Verification items for the finished model (mm, model axes). Face numbers are marked on the shaded views. A direction names the side the tool comes from. Give positions to 0.01 mm unless a question says otherwise; leave off trailing zeros. Write each loop counter-clockwise with the first axis right and the second up, starting at its lowest first coordinate (ties: lowest second). Pieces come first, ordered by that corner, then holes. Notation, with made-up numbers: (35.25, -7.75) - (85.25, -7.75) arc R28 cw to (85.25, 26.25) - close; hole circle Ø11 at (73, 86). An arc over 180 degrees is marked (long way). Put each result on its own line as item: value.
from build123d import *

# Parameters (mm, degrees)
SKETCH_1_R      = 1.05
SKETCH_1_R_2    = 1.5
EXTRUDE_3_DEPTH = 15


with BuildPart() as part:
    # 草图1 → 凸台-拉伸3 (new body)
    with BuildSketch(Plane(origin=(0, 0, 0), x_dir=(1, 0, 0), z_dir=(0, 1, 0))):
        with BuildLine():
            Line((-4.997530566, 2.110812699), (-12.214, 10.272242924))
            Line((-12.214, 10.272242924), (-12.214, 11.219))
            ThreePointArc((-12.214, 11.219), (-11.481766953, 12.986766953), (-9.714, 13.719))
            Line((-9.714, 13.719), (-8.587402673, 13.719))
            Line((-8.587402673, 13.719), (-1.66039255, 5.884932345))
            Line((-1.66039255, 5.884932345), (1.66039255, 5.884932345))
            Line((1.66039255, 5.884932345), (8.587402672, 13.719))
            Line((8.587402672, 13.719), (9.714, 13.719))
            ThreePointArc((9.714, 13.719), (11.481766953, 12.986766953), (12.214, 11.219))
            Line((12.214, 11.219), (12.214, 10.317530105))
            Line((12.214, 10.317530105), (4.997530566, 2.139803462))
            Line((4.997530566, 2.139803462), (4.997530566, -1.644812699))
            Line((4.997530566, -1.644812699), (12.214, -9.806242924))
            Line((12.214, -9.806242924), (12.214, -10.753))
            ThreePointArc((12.214, -10.753), (11.481766953, -12.520766953), (9.714, -13.253))
            Line((9.714, -13.253), (8.587402673, -13.253))
            Line((8.587402673, -13.253), (1.66039255, -5.418932345))
            Line((1.66039255, -5.418932345), (-1.672707789, -5.418932345))
            Line((-1.672707789, -5.418932345), (-8.585913897, -13.253))
            Line((-8.585913897, -13.253), (-9.714, -13.253))
            ThreePointArc((-9.714, -13.253), (-11.481766953, -12.520766953), (-12.214, -10.753))
            Line((-12.214, -10.753), (-12.214, -9.806242924))
            Line((-12.214, -9.806242924), (-4.997530566, -1.644812699))
            Line((-4.997530566, -1.644812699), (-4.997530566, 2.110812699))
        make_face()
        with Locations(Location((-9.714, 11.219, 0), (0, 0, 270))):
            Circle(SKETCH_1_R, mode=Mode.SUBTRACT)
        with Locations(Location((9.714, 11.219, 0), (0, 0, 270))):
            Circle(SKETCH_1_R, mode=Mode.SUBTRACT)
        with Locations(Location((-9.714, -10.753, 0), (0, 0, 270))):
            Circle(SKETCH_1_R, mode=Mode.SUBTRACT)
        with Locations(Location((9.714, -10.753, 0), (0, 0, 270))):
            Circle(SKETCH_1_R, mode=Mode.SUBTRACT)
        with Locations(Location((0, 0, 0), (0, 0, 270))):
            Circle(SKETCH_1_R_2, mode=Mode.SUBTRACT)
    extrude(amount=EXTRUDE_3_DEPTH)


solid = part.part
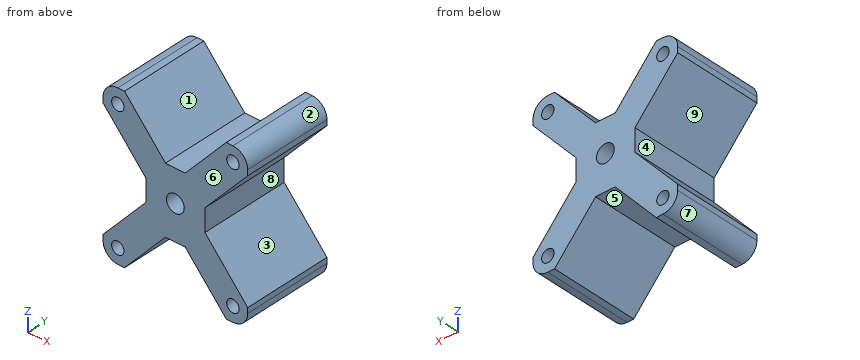
Q1. Section check D-D, the plane x = 10.25. Record the cut outline in (y, z).
Answers follow:
outline: (0, -13.66) - (15, -13.66) - (15, -12.12) - (0, -12.12) - close; (0, -10.32) - (15, -10.32) - (15, -8.09) - (0, -8.09) - close; (0, 7.59) - (15, 7.59) - (15, 9.85) - (0, 9.85) - close; (0, 11.66) - (15, 11.66) - (15, 13.19) - (0, 13.19) - close
Q2. Set-up check for the marked faces 1, 2, 3, 4 and 5: record each of +Z, -Z, +X, -X, +Y, -Y from which the full face is reachable in a straight line by a thin tool's end or side.
Answers follow:
face 1: +Z, +Y, -Y
face 2: +Z, +X, +Y, -Y
face 3: +X, +Y, -Y
face 4: -X, +Y, -Y
face 5: -Z, +Y, -Y
Q3. Release check for a two-part mould opening along Z. For the marked faces 6, 7, 8 and 9 record: released by +Z, released by -Z, zero draft, split by the parting line, or undercut.
Answers follow:
face 6: zero draft
face 7: released by -Z
face 8: undercut
face 9: undercut
Q4. Section check B-B, the plane x = 0. Record the cut outline in (y, z).
Answers follow:
outline: (0, -5.88) - (15, -5.88) - (15, -1.5) - (0, -1.5) - close; (0, 1.5) - (15, 1.5) - (15, 5.42) - (0, 5.42) - close
Q5. Go/stop test with flat-tipped pins: pin 1 Ø3 at (y, z) = (9.5, -0.5) entering from -X; pin 2 Ø2.5 at (x, y) = (0, 10) entering from +Z; pin 3 Ø4 at (y, z) = (5, 0) entering from -X; pin 4 Ø2.5 at (x, z) = (-9.714, -11.219) entering from -Y. Record where each tip stops, or that it passes through.
Answers follow:
pin 1: stops at x = -5
pin 2: stops at z = 5.42
pin 3: stops at x = -5.31
pin 4: stops at y = 0
Q6. Scan lines: line 1 along Z through (x, y) = (9, 4.75); line 2 along X through (y, z) = (7, 0); line 3 along X through (y, z) = (5.5, -11.25). Record each from-to range of solid material in increasing order.
Answers follow:
line 1: z = -13.72 to -11.99, -10.45 to -6.68, 6.17 to 9.98, 11.52 to 13.25
line 2: x = -5 to -1.5, 1.5 to 5
line 3: x = -12.21 to -10.76, -8.66 to -6.4, 6.4 to 8.66, 10.76 to 12.21
Q7. Section check A-A, the plane z = 0. Record the cut outline in (x, y), plus the area to 3 significant figures.
Answers follow:
outline: (-5, 0) - (-1.5, 0) - (-1.5, 15) - (-5, 15) - close; (1.5, 0) - (5, 0) - (5, 15) - (1.5, 15) - close
area: 105 mm2
Q8. Section check C-C, the plane y = 7.25. Give the number of separate pieces and of enclosed holes in the cut face, plus the area to 3 significant figures.
Answers follow:
separate pieces: 1
enclosed holes: 5
area: 300 mm2
